```python
from build123d import *

# Parameters (mm, degrees)
F3_R     = 1.775
F4_DEPTH = 50


with BuildPart() as f1:
    # F0 (on Top) → F1 (revolve)
    with BuildSketch(Plane.XY):
        with BuildLine():
            ThreePointArc((14.057952, 77.55), (1.557952, 72.585443), (-10.942048, 77.55))
            Line((-10.942048, 77.55), (-10.942048, 4.1))
            Line((-10.942048, 4.1), (3.057952, 4.1))
            Line((3.057952, 4.1), (3.057952, 15.1))
            ThreePointArc((3.057952, 15.1), (1.377341, 43.775629), (14.057952, 69.55))
            Line((14.057952, 69.55), (14.057952, 77.55))
        make_face()
    revolve(axis=Axis((3.827849, 0, 0), (1, 0, 0)))

    # F3 (on offset) → F4 (cut)
    with BuildSketch(Plane.YZ.offset(15)):
        with BuildLine():
            ThreePointArc((-49.468369, -42.40974), (-31.529137, -34.888813), (-21.053099, -18.498785))
            ThreePointArc((-21.053099, -18.498785), (-22.917448, -7.44633), (-27.905628, 2.59113))
            ThreePointArc((-27.905628, 2.59113), (-46.014738, 9.693281), (-64.948572, 5.233423))
            ThreePointArc((-64.948572, 5.233423), (-66.894063, 3.38691), (-67.840566, 0.877193))
            ThreePointArc((-67.840566, 0.877193), (-65.842617, -21.393563), (-54.368569, -40.585348))
            ThreePointArc((-54.368569, -40.585348), (-52.127658, -42.059412), (-49.468369, -42.40974))
        make_face()
        with BuildLine():
            ThreePointArc((-55.620627, 33.941885), (-42.924273, 19.204755), (-24.099155, 14.306248))
            ThreePointArc((-24.099155, 14.306248), (-14.163762, 19.494746), (-6.159002, 27.340532))
            ThreePointArc((-6.159002, 27.340532), (-5.000477, 46.758005), (-15.092932, 63.386979))
            ThreePointArc((-15.092932, 63.386979), (-17.450259, 64.666647), (-20.129627, 64.79128))
            ThreePointArc((-20.129627, 64.79128), (-40.692975, 56.009075), (-55.399772, 39.16602))
            ThreePointArc((-55.399772, 39.16602), (-56.10921, 36.579276), (-55.620627, 33.941885))
        make_face()
        with BuildLine():
            ThreePointArc((15.092932, 63.386979), (5.000477, 46.758005), (6.159002, 27.340532))
            ThreePointArc((6.159002, 27.340532), (14.163762, 19.494746), (24.099155, 14.306248))
            ThreePointArc((24.099155, 14.306248), (42.924273, 19.204755), (55.620627, 33.941885))
            ThreePointArc((55.620627, 33.941885), (56.10921, 36.579276), (55.399772, 39.16602))
            ThreePointArc((55.399772, 39.16602), (40.692975, 56.009075), (20.129627, 64.79128))
            ThreePointArc((20.129627, 64.79128), (17.450259, 64.666647), (15.092932, 63.386979))
        make_face()
        with BuildLine():
            ThreePointArc((64.948572, 5.233423), (46.014738, 9.693281), (27.905628, 2.59113))
            ThreePointArc((27.905628, 2.59113), (22.917448, -7.44633), (21.053099, -18.498785))
            ThreePointArc((21.053099, -18.498785), (31.529137, -34.888813), (49.468369, -42.40974))
            ThreePointArc((49.468369, -42.40974), (52.127658, -42.059412), (54.368569, -40.585348))
            ThreePointArc((54.368569, -40.585348), (65.842617, -21.393563), (67.840566, 0.877193))
            ThreePointArc((67.840566, 0.877193), (66.894063, 3.38691), (64.948572, 5.233423))
        make_face()
        with BuildLine():
            ThreePointArc((11.087624, -25.739126), (0, -24.096831), (-11.087624, -25.739126))
            ThreePointArc((-11.087624, -25.739126), (-23.438194, -40.767227), (-25.047493, -60.152546))
            ThreePointArc((-25.047493, -60.152546), (-23.892545, -62.573422), (-21.798148, -64.249144))
            ThreePointArc((-21.798148, -64.249144), (0, -69.231025), (21.798148, -64.249144))
            ThreePointArc((21.798148, -64.249144), (23.892545, -62.573422), (25.047493, -60.152546))
            ThreePointArc((25.047493, -60.152546), (23.438194, -40.767227), (11.087624, -25.739126))
        make_face()
        with Locations((0.254906, 8.229248)):
            Circle(F3_R)
        with Locations((8.304906, 0.179248)):
            Circle(F3_R)
        with Locations((0.254906, -7.870752)):
            Circle(F3_R)
        with Locations((-7.795094, 0.179248)):
            Circle(F3_R)
    extrude(amount=-F4_DEPTH, mode=Mode.SUBTRACT)


solid = f1.part
```
The model under review builds one solid part; all positions refer to its coordinate system, in mm. Round coordinates to 2 decimals unless told otherwise and drop trailing zeros.
(1) Wall thickness on L1, parallel to Z at x = -8.75, y = 18; L2, parallel to Y at x = 1.25, z = 58.5; L3, parallel to Y at x = -7, z = -16: over which ranges is each line inside the solid? List them lowest first.
(2) Insertion check: pin 1 (3 mm diameter, centred on x = -7.5, y = -4.5, fed in from -Z); pin 2 (15 mm diameter, centred on y = -1, z = 0, fed in from +X); pin 3 (3 mm diameter, centred on x = 2, y = 47.5, fed in from +Z); pin 4 (5.5 mm diameter, centred on y = 0.25, z = -7.87, fed in from -X). Each pin has a flat end and moves straight along its axis. Give the tip position at first contact, or say it passes through.
(3) Mouldability with a two-part tool opening along Y and no side actions: class faces 1 (the cylindrical face through (1.012, -52.163, -42.046)), 2 (the flat face through (-10.942, 16, 1)) as +Y half, -Y half, draft (parallel to the pull), parting line (faces both ways), or undercut.
(4) We need section A-A on y = 46. Give the number of separate pieces and of enclosed holes in the cut face, and give its area (3 significant figures).
Findings below:
1. L1: z = -73.61 to -65.89, -31.82 to 17.04, 64.79 to 73.61
1. L2: y = -42.97 to -36.92, -10.58 to 10.58, 36.92 to 42.97
1. L3: y = -72.99 to -67.27, -21.19 to 21.19, 67.27 to 72.99
2. pin 1: stops at z = -75.83
2. pin 2: stops at x = 3.06
2. pin 3: stops at z = 56.16
2. pin 4: stops at x = -10.94
3. face 1: undercut
3. face 2: draft
4. separate pieces: 3
4. enclosed holes: 0
4. area: 699 mm2
